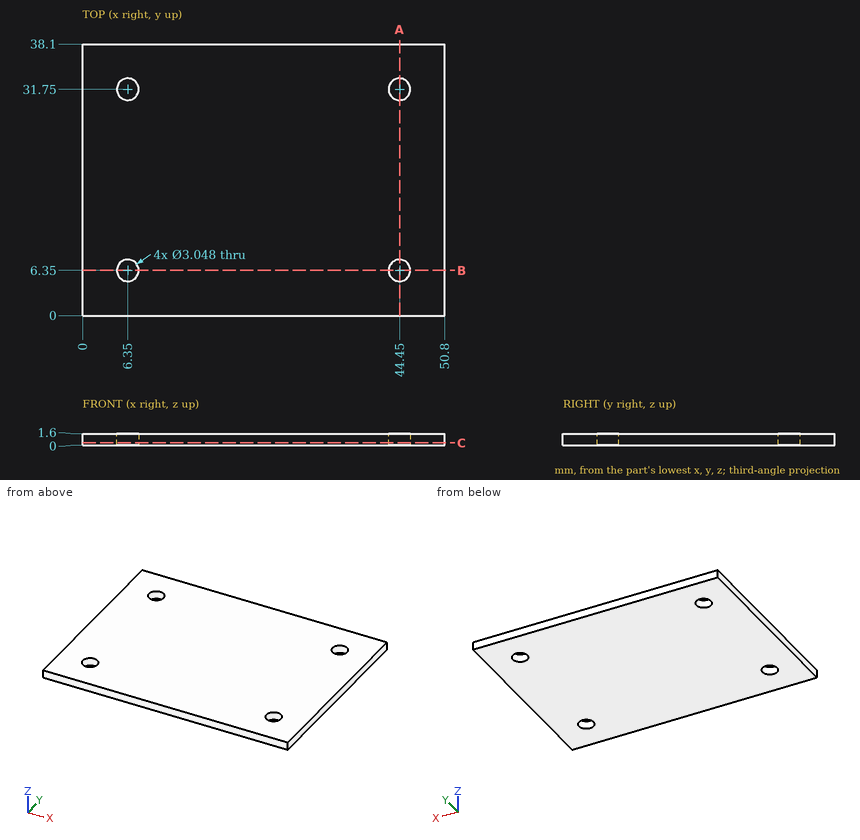
Geometry: see drawing. Coordinates: mm, zero at the bounding-box minimum. Coordinates: 2 decimals unless noted, no trailing zeros. Write each loop counter-clockwise with the first axis right and the second up, starting at its lowest first coordinate (ties: lowest second). Pieces come first, ordered by that corner, then holes. Notation, with made-up numbers: M 62.5,37 L 99.5,37 A11 cw 99.5,45 Z; hole C 17.5,26.5 d5. An arc over 180 degrees is marked long. Answer as a JSON object with one key per item and string values.
1. Ray query, L1, parallel to Y at x = 6.35, z = 0.5; L2, parallel to X at y = 30.5, z = 0.15; L3, parallel to X at y = 5, z = 0.95. Return the intervals inside material, ascending.
Evaluation:
{"L1": "0 to 4.83, 7.87 to 30.23, 33.27 to 38.1", "L2": "0 to 5.48, 7.22 to 43.58, 45.32 to 50.8", "L3": "0 to 5.64, 7.06 to 43.74, 45.16 to 50.8"}
2. Cut plane C-C on z = 0.3. Output: boundary loops of the cut face in (x, y).
Evaluation:
{"outline": "M 0,0 L 50.8,0 L 50.8,38.1 L 0,38.1 Z; hole C 6.35,6.35 d3.05; hole C 6.35,31.75 d3.05; hole C 44.45,6.35 d3.05; hole C 44.45,31.75 d3.05"}
3. Cut plane A-A on x = 44.45. Output: boundary loops of the cut face in (y, z).
Evaluation:
{"outline": "M 0,0 L 4.83,0 L 4.83,1.6 L 0,1.6 Z; M 7.87,0 L 30.23,0 L 30.23,1.6 L 7.87,1.6 Z; M 33.27,0 L 38.1,0 L 38.1,1.6 L 33.27,1.6 Z"}
4. Cut plane B-B on y = 6.35. Output: boundary loops of the cut face in (x, z).
Evaluation:
{"outline": "M 0,0 L 4.83,0 L 4.83,1.6 L 0,1.6 Z; M 7.87,0 L 42.93,0 L 42.93,1.6 L 7.87,1.6 Z; M 45.97,0 L 50.8,0 L 50.8,1.6 L 45.97,1.6 Z"}
